```python
from build123d import *

# Parameters (mm, degrees)
BODY_DEPTH                                          = 200
AESTHETIC_CHAMFER_SIZE                              = 0.15
CBORE_FOR_M4_HEX_SOCKET_HEAD_CAP_SCREW1_D           = 4.5
CBORE_FOR_M4_HEX_SOCKET_HEAD_CAP_SCREW1_CBORE_D     = 8
CBORE_FOR_M4_HEX_SOCKET_HEAD_CAP_SCREW1_CBORE_DEPTH = 3.2
LPATTERN1_COUNT                                     = 4
LPATTERN1_PITCH                                     = 60


with BuildPart() as part:
    # Rail Profile → Body (new body)
    with BuildSketch(Plane.XY):
        with BuildLine():
            Line((-7, 0), (7, 0))
            Line((7, 0), (7.5, 0.5))
            Line((7.5, 0.5), (7.5, 3.085786438))
            ThreePointArc((7.5, 3.085786438), (7.423879533, 3.46846987), (7.207106781, 3.792893219))
            Line((7.207106781, 3.792893219), (4.867157288, 6.132842712))
            ThreePointArc((4.867157288, 6.132842712), (4.780448187, 6.262612052), (4.75, 6.415685425))
            Line((4.75, 6.415685425), (4.75, 8.584314575))
            ThreePointArc((4.75, 8.584314575), (4.780448187, 8.737387948), (4.867157288, 8.867157288))
            Line((4.867157288, 8.867157288), (5.062965362, 9.062965362))
            ThreePointArc((5.062965362, 9.062965362), (5.134996734, 9.161242682), (5.17409812, 9.27664646))
            ThreePointArc((5.17409812, 9.27664646), (5.61862915, 10.13137085), (6.47335354, 10.57590188))
            ThreePointArc((6.47335354, 10.57590188), (6.694124352, 10.694306692), (6.801170165, 10.920803148))
            ThreePointArc((6.801170165, 10.920803148), (6.915305692, 11.154571658), (7.149074202, 11.268707185))
            ThreePointArc((7.149074202, 11.268707185), (7.399691242, 11.400760606), (7.5, 11.665685425))
            Line((7.5, 11.665685425), (7.5, 12.334314575))
            ThreePointArc((7.5, 12.334314575), (7.399691242, 12.599239394), (7.149074202, 12.731292815))
            ThreePointArc((7.149074202, 12.731292815), (6.915305692, 12.845428342), (6.801170165, 13.079196852))
            ThreePointArc((6.801170165, 13.079196852), (6.694124352, 13.305693308), (6.47335354, 13.42409812))
            ThreePointArc((6.47335354, 13.42409812), (5.61862915, 13.86862915), (5.17409812, 14.72335354))
            ThreePointArc((5.17409812, 14.72335354), (5.134996734, 14.838757318), (5.062965362, 14.937034638))
            Line((5.062965362, 14.937034638), (5, 15))
            Line((5, 15), (-5, 15))
            Line((-5, 15), (-5.062965362, 14.937034638))
            ThreePointArc((-5.062965362, 14.937034638), (-5.134996734, 14.838757318), (-5.17409812, 14.72335354))
            ThreePointArc((-5.17409812, 14.72335354), (-5.61862915, 13.86862915), (-6.47335354, 13.42409812))
            ThreePointArc((-6.47335354, 13.42409812), (-6.694124352, 13.305693308), (-6.801170165, 13.079196852))
            ThreePointArc((-6.801170165, 13.079196852), (-6.915305692, 12.845428342), (-7.149074202, 12.731292815))
            ThreePointArc((-7.149074202, 12.731292815), (-7.399691242, 12.599239394), (-7.5, 12.334314575))
            Line((-7.5, 12.334314575), (-7.5, 11.665685425))
            ThreePointArc((-7.5, 11.665685425), (-7.399691242, 11.400760606), (-7.149074202, 11.268707185))
            ThreePointArc((-7.149074202, 11.268707185), (-6.915305692, 11.154571658), (-6.801170165, 10.920803148))
            ThreePointArc((-6.801170165, 10.920803148), (-6.694124352, 10.694306692), (-6.47335354, 10.57590188))
            ThreePointArc((-6.47335354, 10.57590188), (-5.61862915, 10.13137085), (-5.17409812, 9.27664646))
            ThreePointArc((-5.17409812, 9.27664646), (-5.134996734, 9.161242682), (-5.062965362, 9.062965362))
            Line((-5.062965362, 9.062965362), (-4.867157288, 8.867157288))
            ThreePointArc((-4.867157288, 8.867157288), (-4.780448187, 8.737387948), (-4.75, 8.584314575))
            Line((-4.75, 8.584314575), (-4.75, 6.415685425))
            ThreePointArc((-4.75, 6.415685425), (-4.780448187, 6.262612052), (-4.867157288, 6.132842712))
            Line((-4.867157288, 6.132842712), (-7.207106781, 3.792893219))
            ThreePointArc((-7.207106781, 3.792893219), (-7.423879533, 3.46846987), (-7.5, 3.085786438))
            Line((-7.5, 3.085786438), (-7.5, 0.5))
            Line((-7.5, 0.5), (-7, 0))
        make_face()
    extrude(amount=-BODY_DEPTH)

    # Aesthetic Chamfer
    aesthetic_chamfer_edges = [part.edges().sort_by_distance(p)[0] for p in [
        (7.423879533, 3.46846987, -200),
        (-5.134996734, 9.161242682, -200),
        (-4.965061325, 8.965061325, -200),
        (-4.780448187, 8.737387948, -200),
        (-4.75, 7.5, -200),
        (-4.780448187, 6.262612052, -200),
        (-6.037132034, 4.962867966, -200),
        (-7.423879533, 3.46846987, -200),
        (-7.5, 1.792893219, -200),
        (-7.25, 0.25, -200),
        (0, 0, -200),
        (6.037132034, 4.962867966, -200),
        (4.780448187, 6.262612052, -200),
        (4.75, 7.5, -200),
        (4.780448187, 8.737387948, -200),
        (4.965061325, 8.965061325, -200),
        (5.134996734, 9.161242682, -200),
        (5.61862915, 10.13137085, -200),
        (6.694124352, 10.694306692, -200),
        (0, 0, 0),
        (-7.25, 0.25, 0),
        (-7.5, 1.792893219, 0),
        (-7.423879533, 3.46846987, 0),
        (-6.037132034, 4.962867966, 0),
        (-4.780448187, 6.262612052, 0),
        (6.915305692, 11.154571658, -200),
        (-4.75, 7.5, 0),
        (-4.780448187, 8.737387948, 0),
        (-4.965061325, 8.965061325, 0),
        (-5.134996734, 9.161242682, 0),
        (-5.61862915, 10.13137085, 0),
        (-6.694124352, 10.694306692, 0),
        (-6.915305692, 11.154571658, 0),
        (7.25, 0.25, -200),
        (7.399691242, 11.400760606, -200),
        (-7.399691242, 11.400760606, 0),
        (-7.5, 12, 0),
        (-7.399691242, 12.599239394, 0),
        (-6.915305692, 12.845428342, 0),
        (-6.694124352, 13.305693308, 0),
        (-5.61862915, 13.86862915, 0),
        (-5.134996734, 14.838757318, 0),
        (-5.031482681, 14.968517319, 0),
        (7.5, 12, -200),
        (0, 15, 0),
        (5.031482681, 14.968517319, 0),
        (5.134996734, 14.838757318, 0),
        (5.61862915, 13.86862915, 0),
        (6.694124352, 13.305693308, 0),
        (6.915305692, 12.845428342, 0),
        (7.399691242, 12.599239394, 0),
        (7.399691242, 12.599239394, -200),
        (7.5, 12, 0),
        (7.399691242, 11.400760606, 0),
        (6.915305692, 11.154571658, 0),
        (6.694124352, 10.694306692, 0),
        (5.61862915, 10.13137085, 0),
        (5.134996734, 9.161242682, 0),
        (4.965061325, 8.965061325, 0),
        (4.780448187, 8.737387948, 0),
        (6.915305692, 12.845428342, -200),
        (4.75, 7.5, 0),
        (4.780448187, 6.262612052, 0),
        (6.037132034, 4.962867966, 0),
        (7.423879533, 3.46846987, 0),
        (7.5, 1.792893219, 0),
        (7.25, 0.25, 0),
        (6.694124352, 13.305693308, -200),
        (5.61862915, 13.86862915, -200),
        (5.134996734, 14.838757318, -200),
        (5.031482681, 14.968517319, -200),
        (0, 15, -200),
        (-5.031482681, 14.968517319, -200),
        (7.5, 1.792893219, -200),
        (-5.134996734, 14.838757318, -200),
        (-5.61862915, 13.86862915, -200),
        (-6.694124352, 13.305693308, -200),
        (-6.915305692, 12.845428342, -200),
        (-7.399691242, 12.599239394, -200),
        (-7.5, 12, -200),
        (-7.399691242, 11.400760606, -200),
        (-6.915305692, 11.154571658, -200),
        (-6.694124352, 10.694306692, -200),
        (-5.61862915, 10.13137085, -200),
    ]]
    chamfer(aesthetic_chamfer_edges, length=AESTHETIC_CHAMFER_SIZE)

    # CBORE for M4 Hex Socket Head Cap Screw1 (through all)
    with Locations(Plane(origin=(0, 15, 0), x_dir=(1, 0, 0), z_dir=(0, 1, 0))):
        with Locations((0, 10)):
            cbore_for_m4_hex_socket_head_cap_screw1 = CounterBoreHole(CBORE_FOR_M4_HEX_SOCKET_HEAD_CAP_SCREW1_D / 2, CBORE_FOR_M4_HEX_SOCKET_HEAD_CAP_SCREW1_CBORE_D / 2, CBORE_FOR_M4_HEX_SOCKET_HEAD_CAP_SCREW1_CBORE_DEPTH)

    # LPattern1: CBORE for M4 Hex Socket Head Cap Screw1 ×4
    with Locations(*[(0, 0, -i * LPATTERN1_PITCH) for i in range(1, LPATTERN1_COUNT)]):
        add(cbore_for_m4_hex_socket_head_cap_screw1, mode=Mode.SUBTRACT)


solid = part.part
```
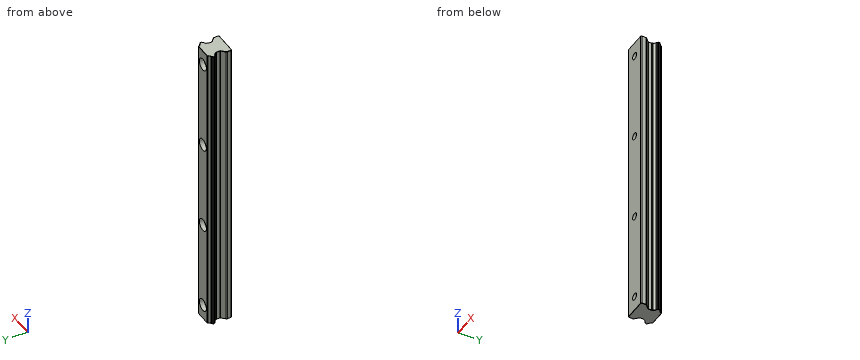
The listing builds one solid part. Answer for the finished solid, in the listing's coordinates (mm). Coordinates: 2 decimals unless noted, no trailing zeros. Answer as a JSON object with one key per item and string values. Group by question number.
1. Section A-A on x = 0 is taken. State how many separate pieces and enclosed holes the cut face has, then the cut area to 3 significant figures.
2. Flat-ended cylindrical pins translate along their axes: P1, Ø1.1, axis at y = 8, z = -143.5, coming from the +X side; P2, Ø2.5, axis at y = 8, z = -58, coming from the -X side; P3, Ø2.5, axis at x = 2, z = -188.5, coming from the +Y side; P4, Ø3.5, axis at x = 0, z = -70, coming from the -Y side. Find the tip coordinate at first contact, or state that the pin passes through.
3. Straight lines are drawn through the part: line 1 (Z direction, x = 0, y = 12.85); line 2 (Z direction, x = 0, y = 6.75); line 3 (X direction, y = 13.05, z = -190). For each, find the intervals that lie inside material, in ascending order.
Values follow:
{
 "1": {"separate pieces": "5", "enclosed holes": "0", "area": "2,690 mm2"},
 "2": {"P1": "x = 4.75", "P2": "x = -5.17", "P3": "y = 11.8", "P4": "through"},
 "3": {"line 1": "-200 to -194, -186 to -134, -126 to -74, -66 to -14, -6 to 0", "line 2": "-200 to -192.25, -187.75 to -132.25, -127.75 to -72.25, -67.75 to -12.25, -7.75 to 0", "line 3": "-6.81 to -4, 4 to 6.81"}
}
